```python
from build123d import *

# Parameters (mm, degrees)
F0_W         = 78.3775448799
F0_H         = 75.6465569139
F1_DEPTH     = 25
F2_R         = 12.0203528279
F3_DEPTH     = 49.9
F4_T         = -2.5
F5_R         = 6.6018014855
F6_DEPTH     = 25
F7_T         = 2.5
F7_T3_DEPTH  = 27.5
F7_T5_DEPTH  = 78.3775448799
F7_T7_DEPTH  = 75.6465569139
F8_DEPTH     = 25
F9_R         = 7.0468826158
F10_DEPTH    = 25
F11_T        = 2.5
F11_T3_DEPTH = 27.5
F11_T5_DEPTH = 78.3775448799
F11_T7_DEPTH = 75.6465569139
F12_DEPTH    = 25
F13_W        = 42.1091411263
F13_H        = 4.6861004084
F14_DEPTH    = 25
F15_W        = 78.3775448799
F15_H        = 75.6465569139
F16_DEPTH    = 15
F17_R        = 10.5957056812
F18_DEPTH    = 25
F19_DEPTH    = 25
F20_DEPTH    = 25
F21_DEPTH    = 25


# Not quite as in the source:
# - a shell that OpenCascade refuses in one call is made with other operations: the cavity is built on its own and cut out


with BuildPart() as f1:
    # F0 (on Top) → F1 (new body)
    with BuildSketch(Plane.XY):
        Rectangle(F0_W, F0_H)
    extrude(amount=F1_DEPTH)

    # F2 (on face) → F3 (cut)
    with BuildSketch(Plane(origin=(0, 0, 0), x_dir=(1, 0, 0), z_dir=(0, 0, -1))):
        Circle(F2_R)
    extrude(amount=-F3_DEPTH, mode=Mode.SUBTRACT)

    # F4
    f4_openings = [f1.faces().sort_by_distance(p)[0] for p in [
        (0, 36.733992, 0),
    ]]
    offset(amount=F4_T, openings=f4_openings)

    # F5 (on face) → F6 (join)
    with BuildSketch(Plane(origin=(0, 0, 22.5), x_dir=(1, 0, 0), z_dir=(0, 0, -1))):
        with Locations((-26.0466337204, 26.645489037)):
            Circle(F5_R)
    extrude(amount=F6_DEPTH)

    # F7: shell of thickness 2.5, made by hand


with BuildPart() as f7_core1:
    # F7_t2: copy of F1
    add(f1.part)

    # the walls: a layer under each face that stays
    f7_faces = [f7_core1.faces().sort_by_distance(p)[0] for p in [
        (0, 37.8232784569, 12.5),
        (39.18877244, 0, 12.5),
        (-39.18877244, 0, 12.5),
        (-36.7394741625, 7.0043108254, 0),
        (-26.1258482933, -25.2155189713, 25),
        (0, -37.8232784569, 12.5),
        (0, 35.3232784569, 11.25),
        (36.68877244, 0, 11.25),
        (0, -35.3232784569, 11.25),
        (-36.68877244, 0, 11.25),
        (-12.0203528279, 0, 12.5),
        (-24.4591816266, 0, 22.5),
        (-9.6802352186, -9.6802352186, 0),
        (-32.6484352059, -26.645489037, 10),
        (-14.5203528279, 0, 11.25),
    ]]
    thicken(f7_faces, amount=-F7_T, mode=Mode.SUBTRACT)

    # F7_s4 → F7_t3 (cut)
    with BuildSketch(Plane.XY.offset(-2.5)):
        Polygon((36.66377244, 35.2982784569), (36.68877244, 37.8232784569), (39.18877244, 37.8232784569), (39.18877244, 35.3232784569), align=None)
        Polygon((-36.66377244, 35.2982784569), (-36.68877244, 37.8232784569), (-39.18877244, 37.8232784569), (-39.18877244, 35.3232784569), align=None)
        Polygon((36.66377244, -35.2982784569), (39.18877244, -35.3232784569), (39.18877244, -37.8232784569), (36.68877244, -37.8232784569), align=None)
        Polygon((-36.66377244, -35.2982784569), (-36.68877244, -37.8232784569), (-39.18877244, -37.8232784569), (-39.18877244, -35.3232784569), align=None)
    extrude(amount=F7_T3_DEPTH, mode=Mode.SUBTRACT)

    # F7_s6 → F7_t5 (cut)
    with BuildSketch(Plane.YZ.offset(-39.18877244)):
        Polygon((35.2982784569, 22.475), (37.8232784569, 22.5), (37.8232784569, 25), (35.3232784569, 25), align=None)
        Polygon((-35.2982784569, 22.475), (-37.8232784569, 22.5), (-37.8232784569, 25), (-35.3232784569, 25), align=None)
    extrude(amount=F7_T5_DEPTH, mode=Mode.SUBTRACT)

    # F7_s8 → F7_t7 (cut)
    with BuildSketch(Plane.XZ.offset(-37.8232784569)):
        Polygon((36.66377244, 22.475), (39.18877244, 22.5), (39.18877244, 25), (36.68877244, 25), align=None)
        Polygon((-36.66377244, 22.475), (-39.18877244, 22.5), (-39.18877244, 25), (-36.68877244, 25), align=None)
    extrude(amount=F7_T7_DEPTH, mode=Mode.SUBTRACT)

    # F7_s9 → F7_t10 (revolve, cut)
    with BuildSketch(Plane.XZ.offset(26.645489037)):
        Polygon((-19.4198322349, 22.475), (-19.4448322349, 25), (-21.9448322349, 25), (-21.9448322349, 22.5), align=None)
    revolve(axis=Axis((-26.0466337204, -26.645489037, 22.5), (0, 0, -1)), mode=Mode.SUBTRACT)

    # F7_s11 → F7_t12 (revolve, cut)
    with BuildSketch(Plane.XZ):
        Polygon((14.5453528279, 22.475), (14.5203528279, 25), (12.0203528279, 25), (12.0203528279, 22.5), align=None)
    revolve(axis=Axis((0, 0, 22.5), (0, 0, -1)), mode=Mode.SUBTRACT)


with BuildPart() as f1_1:
    add(f1.part)

    # what is left inside the walls is the cavity
    f7_cavity = [f7_core1.part.solids().sort_by_distance(p)[0] for p in [
        (-30.123435, -26.645489, 5.833333),
    ]]
    add(f7_cavity, mode=Mode.SUBTRACT)

    # F8 (cut): a face of the model
    f8_faces = [f1_1.faces().sort_by_distance(p)[0] for p in [
        (-26.0466337204, -26.645489037, 22.5),
    ]]
    extrude(f8_faces, amount=-F8_DEPTH, mode=Mode.SUBTRACT)

    # F9 (on face) → F10 (join)
    with BuildSketch(Plane(origin=(0, 0, 22.5), x_dir=(1, 0, 0), z_dir=(0, 0, -1))):
        with Locations((26.8326979131, 27.2501390427)):
            Circle(F9_R)
    extrude(amount=F10_DEPTH)

    # F11: shell of thickness 2.5, made by hand


with BuildPart() as f11_core1:
    # F11_t2: copy of F1
    add(f1_1.part)

    # the walls: a layer under each face that stays
    f11_faces = [f11_core1.faces().sort_by_distance(p)[0] for p in [
        (0, 37.8232784569, 12.5),
        (39.18877244, 0, 12.5),
        (-39.18877244, 0, 12.5),
        (-36.7394741625, 7.0043108254, 0),
        (-26.1258482933, 0, 25),
        (0, -37.8232784569, 12.5),
        (0, 35.3232784569, 11.25),
        (36.68877244, 0, 11.25),
        (0, -35.3232784569, 11.25),
        (-36.68877244, 0, 11.25),
        (-30.1484352059, -26.645489037, 23.75),
        (-12.0203528279, 0, 12.5),
        (-24.4591816266, 0, 22.5),
        (-30.1484352059, -26.645489037, 10),
        (-9.6802352186, -9.6802352186, 0),
        (-32.6484352059, -26.645489037, 10),
        (19.7858152973, -27.2501390427, 10),
        (-14.5203528279, 0, 11.25),
        (-30.4478347107, -22.2442880467, -2.5),
    ]]
    thicken(f11_faces, amount=-F11_T, mode=Mode.SUBTRACT)

    # F11_s4 → F11_t3 (cut)
    with BuildSketch(Plane.XY.offset(-2.5)):
        Polygon((36.66377244, 35.2982784569), (36.68877244, 37.8232784569), (39.18877244, 37.8232784569), (39.18877244, 35.3232784569), align=None)
        Polygon((-36.66377244, 35.2982784569), (-36.68877244, 37.8232784569), (-39.18877244, 37.8232784569), (-39.18877244, 35.3232784569), align=None)
        Polygon((36.66377244, -35.2982784569), (39.18877244, -35.3232784569), (39.18877244, -37.8232784569), (36.68877244, -37.8232784569), align=None)
        Polygon((-36.66377244, -35.2982784569), (-36.68877244, -37.8232784569), (-39.18877244, -37.8232784569), (-39.18877244, -35.3232784569), align=None)
    extrude(amount=F11_T3_DEPTH, mode=Mode.SUBTRACT)

    # F11_s6 → F11_t5 (cut)
    with BuildSketch(Plane.YZ.offset(-39.18877244)):
        Polygon((35.2982784569, 22.475), (37.8232784569, 22.5), (37.8232784569, 25), (35.3232784569, 25), align=None)
        Polygon((-35.2982784569, 22.475), (-37.8232784569, 22.5), (-37.8232784569, 25), (-35.3232784569, 25), align=None)
    extrude(amount=F11_T5_DEPTH, mode=Mode.SUBTRACT)

    # F11_s8 → F11_t7 (cut)
    with BuildSketch(Plane.XZ.offset(-37.8232784569)):
        Polygon((36.66377244, 22.475), (39.18877244, 22.5), (39.18877244, 25), (36.68877244, 25), align=None)
        Polygon((-36.66377244, 22.475), (-39.18877244, 22.5), (-39.18877244, 25), (-36.68877244, 25), align=None)
    extrude(amount=F11_T7_DEPTH, mode=Mode.SUBTRACT)

    # F11_s9 → F11_t10 (revolve, cut)
    with BuildSketch(Plane.XZ.offset(26.645489037)):
        Polygon((-19.4198322349, 22.475), (-19.4448322349, 25), (-21.9448322349, 25), (-21.9448322349, 22.5), align=None)
    revolve(axis=Axis((-26.0466337204, -26.645489037, 22.5), (0, 0, -1)), mode=Mode.SUBTRACT)

    # F11_s11 → F11_t12 (revolve, cut)
    with BuildSketch(Plane.XZ.offset(27.2501390427)):
        Polygon((33.9045805288, 22.475), (33.8795805288, 25), (31.3795805288, 25), (31.3795805288, 22.5), align=None)
    revolve(axis=Axis((26.8326979131, -27.2501390427, 22.5), (0, 0, -1)), mode=Mode.SUBTRACT)

    # F11_s13 → F11_t14 (revolve, cut)
    with BuildSketch(Plane.XZ):
        Polygon((14.5453528279, 22.475), (14.5203528279, 25), (12.0203528279, 25), (12.0203528279, 22.5), align=None)
    revolve(axis=Axis((0, 0, 22.5), (0, 0, -1)), mode=Mode.SUBTRACT)


with BuildPart() as f1_2:
    add(f1_1.part)

    # what is left inside the walls is the cavity
    f11_cavity = [f11_core1.part.solids().sort_by_distance(p)[0] for p in [
        (22.310815, -27.250139, 5.833333),
    ]]
    add(f11_cavity, mode=Mode.SUBTRACT)

    # F12 (cut): a face of the model
    f12_faces = [f1_2.faces().sort_by_distance(p)[0] for p in [
        (26.8326979131, -27.2501390427, 22.5),
    ]]
    extrude(f12_faces, amount=-F12_DEPTH, mode=Mode.SUBTRACT)

    # F13 (on face) → F14 (cut)
    with BuildSketch(Plane.XZ.offset(37.8232784569)):
        with Locations((-0.3970777616, 11.9879292324)):
            Rectangle(F13_W, F13_H)
    extrude(amount=-F14_DEPTH, mode=Mode.SUBTRACT)

    # F15 (on face) → F16 (join)
    with BuildSketch(Plane(origin=(0, 0, 0), x_dir=(1, 0, 0), z_dir=(0, 0, -1))):
        Rectangle(F15_W, F15_H)
    extrude(amount=F16_DEPTH)

    # F17 (on face) → F18 (cut)
    with BuildSketch(Plane(origin=(0, 0, -15), x_dir=(1, 0, 0), z_dir=(0, 0, -1))):
        with Locations((-27.1771177649, 22.4702265114)):
            Circle(F17_R)
    extrude(amount=F18_DEPTH, mode=Mode.SUBTRACT)

    # F19 (cut): a face of the model
    f19_faces = [f1_2.faces().sort_by_distance(p)[0] for p in [
        (0, 0, 0),
    ]]
    extrude(f19_faces, amount=-F19_DEPTH, mode=Mode.SUBTRACT)

    # F20 (cut): a face of the model
    f20_faces = [f1_2.faces().sort_by_distance(p)[0] for p in [
        (-26.0466337204, -26.645489037, 0),
    ]]
    extrude(f20_faces, amount=-F20_DEPTH, mode=Mode.SUBTRACT)

    # F21 (cut): a face of the model
    f21_faces = [f1_2.faces().sort_by_distance(p)[0] for p in [
        (26.8326979131, -27.2501390427, 0),
    ]]
    extrude(f21_faces, amount=-F21_DEPTH, mode=Mode.SUBTRACT)


solid = f1_2.part
```
The listing builds one solid part. Answer for the finished solid, in the listing's coordinates (mm). A direction names the side the tool comes from. Round coordinates to 2 decimals unless told otherwise and drop trailing zeros. Write each loop counter-clockwise with the first axis right and the second up, starting at its lowest first coordinate (ties: lowest second). Pieces come first, ordered by that corner, then holes. Notation, with made-up numbers: (26, 57) -> (74, 57) arc R22 ccw to (74, 83) -> close; hole circle Ø9 at (47.5, 78.5). An arc over 180 degrees is marked (long way). Use CSV: the item, a comma, the result in double quotes. Start each with the question number.
(1) Consider L1, parallel to X at y = 0, z = 10; L2, parallel to X at y = 0, z = -9.5; L3, parallel to Z at x = -18, y = -27. Determine where each line is inside the solid, lowest interval first. Write a range as from..to.
(2) Section D-D on y = 24 is taken. Give the vertices of the cut face in (x, z).
(3) Which of the six approach directions +Z, -Z, +X, -X, +Y, -Y give full straight-line access (tool end or side, diameter ignored) to faces 1 (the face through (-1, 37.823, 5)), 2 (the face through (-32.64, -26.94, 11.41)), 3 (the face through (-21.452, -37, 12))?
(4) Each of these flat-tipped pins is pushed along its axis until it touches: pin 1 (19 mm diameter, centred on x = 0, y = 0, fed in from +Z); pin 2 (2.5 mm diameter, centred on x = -2, z = 13, fed in from -Y). Where does it stop, or does it pass through?
(5) Section A-A on y = 0 is taken. Give the vertices of the cut face in (x, z).
(6) The mould has two halves that part along Y. Classify faces 4 (the face through (-1, 35.323, 11)), 5 (the face through (-1, -37, 14.331)), 6 (the face through (-1, -37.823, 5)): released by +Y, released by -Y, zero draft, split by the parting line, or undercut.
(7) Section B-B on x = 0 is taken. Give the vertices of the cut face in (y, z).
(8) Section C-C on z = 1 is taken. Give the vertices of the cut face in (x, y).
A:
1,L1,"x = -39.19..-36.69, -14.52..-12.02, 12.02..14.52, 36.69..39.19"
1,L2,"x = -39.19..-12.02, 12.02..39.19"
1,L3,"z = -15..0, 22.5..25"
2,outline,"(-39.19, -15) -> (39.19, -15) -> (39.19, 25) -> (-39.19, 25) -> close; hole (-36.69, 0) -> (36.69, 0) -> (36.69, 22.5) -> (-36.69, 22.5) -> close"
3,face 1,"+Z, -Z, +X, -X, +Y"
3,face 2,"none"
3,face 3,"-Y"
4,pin 1,"passes through"
4,pin 2,"stops at y = -12.82"
5,outline,"(-39.19, -15) -> (-12.02, -15) -> (-12.02, 25) -> (-39.19, 25) -> close; (12.02, -15) -> (39.19, -15) -> (39.19, 25) -> (12.02, 25) -> close; hole (-36.69, 0) -> (-14.52, 0) -> (-14.52, 22.5) -> (-36.69, 22.5) -> close; hole (14.52, 0) -> (36.69, 0) -> (36.69, 22.5) -> (14.52, 22.5) -> close"
6,face 4,"undercut"
6,face 5,"zero draft"
6,face 6,"released by -Y"
7,outline,"(-37.82, -15) -> (-12.02, -15) -> (-12.02, 25) -> (-37.82, 25) -> (-37.82, 14.33) -> (-35.32, 14.33) -> (-35.32, 22.5) -> (-14.52, 22.5) -> (-14.52, 14.33) -> (-12.82, 14.33) -> (-12.82, 9.64) -> (-14.52, 9.64) -> (-14.52, 0) -> (-35.32, 0) -> (-35.32, 9.64) -> (-37.82, 9.64) -> close; (12.02, -15) -> (37.82, -15) -> (37.82, 25) -> (12.02, 25) -> close; hole (14.52, 0) -> (35.32, 0) -> (35.32, 22.5) -> (14.52, 22.5) -> close"
8,outline,"(-39.19, -37.82) -> (39.19, -37.82) -> (39.19, 37.82) -> (-39.19, 37.82) -> close; circle Ø13.2 at (-26.05, -26.65); circle Ø29.04 at (0, 0); circle Ø14.09 at (26.83, -27.25); hole (-36.69, -35.32) -> (36.69, -35.32) -> (36.69, 35.32) -> (-36.69, 35.32) -> close; hole circle Ø8.2 at (-26.05, -26.65); hole circle Ø24.04 at (0, 0); hole circle Ø9.09 at (26.83, -27.25)"
